Autodesk Inventor part; units mm, degrees
ref_plane "YZ Plane" through (0, 0, 0) normal (1, 0, 0) x (0, 1, 0)
ref_plane "XZ Plane" through (0, 0, 0) normal (0, 1, 0) x (-1, 0, 0)
ref_plane "XY Plane" through (0, 0, 0) normal (0, 0, 1) x (1, 0, 0)
sketch "Sketch1" plane through (0, 0, 0) normal (0, 0, 1) x (1, 0, 0)
  line L0 (0, 0) -> (161.925, 0)
  line L1 (161.925, 0) -> (161.925, 133.35)
  line L2 (161.925, 133.35) -> (0, 133.35)
  line L3 (0, 133.35) -> (0, 0)
  dimension "d0" = 161.925
  dimension "d1" = 133.35
extrude "Extrusion1" add sketch "Sketch1" along normal blind 3.175
sketch "Sketch6" plane through (0, 0, 0) normal (0, 0, -1) x (-1, 0, 0)
  circle A0 centre (-155.575, 122.2375) radius 1.5875
  circle A1 centre (-6.35, 122.2375) radius 1.5875
  circle A2 centre (-155.575, 25.4) radius 1.5875
  circle A3 centre (-6.35, 25.4) radius 1.5875
extrude "Extrusion6" cut sketch "Sketch6" against normal blind 3.175
sketch "Sketch7" plane through (0, 0, 3.175) normal (0, 0, 1) x (1, 0, 0)
  circle A0 centre (155.575, 122.2375) radius 1.5875
  circle A1 centre (6.35, 122.2375) radius 1.5875
  line L0 (9.5885, 120.3678) -> (6.35, 118.498)
  line L1 (6.35, 118.498) -> (3.1115, 120.3678)
  line L2 (3.1115, 120.3678) -> (3.1115, 124.1072)
  line L3 (3.1115, 124.1072) -> (6.35, 125.977)
  line L4 (6.35, 125.977) -> (9.5885, 124.1072)
  line L5 (9.5885, 124.1072) -> (9.5885, 120.3678)
  line L6 (158.8135, 120.3678) -> (155.575, 118.498)
  line L7 (155.575, 118.498) -> (152.3365, 120.3678)
  line L8 (152.3365, 120.3678) -> (152.3365, 124.1072)
  line L9 (152.3365, 124.1072) -> (155.575, 125.977)
  line L10 (155.575, 125.977) -> (158.8135, 124.1072)
  line L11 (158.8135, 124.1072) -> (158.8135, 120.3678)
  circle A2 centre (155.575, 25.4) radius 1.5875
  circle A3 centre (6.35, 25.4) radius 1.5875
  line L12 (9.5885, 23.5303) -> (6.35, 21.6605)
  line L13 (6.35, 21.6605) -> (3.1115, 23.5303)
  line L14 (3.1115, 23.5303) -> (3.1115, 27.2697)
  line L15 (3.1115, 27.2697) -> (6.35, 29.1395)
  line L16 (6.35, 29.1395) -> (9.5885, 27.2697)
  line L17 (9.5885, 27.2697) -> (9.5885, 23.5303)
  line L18 (158.8135, 23.5303) -> (155.575, 21.6605)
  line L19 (155.575, 21.6605) -> (152.3365, 23.5303)
  line L20 (152.3365, 23.5303) -> (152.3365, 27.2697)
  line L21 (152.3365, 27.2697) -> (155.575, 29.1395)
  line L22 (155.575, 29.1395) -> (158.8135, 27.2697)
  line L23 (158.8135, 27.2697) -> (158.8135, 23.5303)
  point P0 (9.5885, 122.2375)
  point P1 (158.8135, 122.2375)
extrude "Extrusion7" cut sketch "Sketch7" against normal blind 1.5875
sketch "Sketch11" plane through (0, 0, 3.175) normal (0, 0, 1) x (1, 0, 0)
  line L0 (161.925, 0) -> (161.925, 133.35)
  line L1 (0, 133.35) -> (0, 0)
  line L2 (0, 102.616) -> (161.925, 102.616)
  line L3 (0, 89.408) -> (161.925, 89.408)
  line L4 (0, 97.79) -> (161.925, 97.79)
  line L5 (0, 94.234) -> (161.925, 94.234)
  line L6 (0, 4.826) -> (161.925, 4.826)
  line L7 (0, 8.382) -> (161.925, 8.382)
  line L8 (0, 0) -> (161.925, 0)
  line L9 (0, 13.208) -> (161.925, 13.208)
  line L10 (0, 47.625) -> (161.925, 47.625)
  line L11 (0, 34.417) -> (161.925, 34.417)
  line L12 (0, 42.799) -> (161.925, 42.799)
  line L13 (0, 39.243) -> (161.925, 39.243)
  line L14 (161.925, 133.35) -> (0, 133.35)
  dimension "d83" = 4.826
  dimension "d84" = 3.556
  dimension "d85" = 4.826
  dimension "d86" = 4.826
  dimension "d87" = 3.556
  dimension "d88" = 4.826
  dimension "d89" = 4.826
  dimension "d90" = 3.556
  dimension "d91" = 4.826
  dimension "d96" = 30.861
  dimension "d98" = 35.56
extrude "Extrusion10" add sketch "Sketch11" along normal blind 3.302 contours L8 L1 L6 L0 | L7 L1 L9 L0 | L11 L1 L13 L0 | L12 L1 L10 L0 | L3 L1 L5 L0 | L4 L1 L2 L0
sketch "Sketch15" plane through (0, 0, 3.175) normal (0, 0, 1) x (1, 0, 0)
  line L0 (0, 102.616) -> (161.925, 102.616)
  line L1 (12.7, 120.65) -> (149.225, 120.65)
  line L2 (149.225, 120.65) -> (149.225, 102.616)
  line L3 (149.225, 102.616) -> (12.7, 102.616)
  line L4 (12.7, 102.616) -> (12.7, 120.65)
  point P0 (0, 0)
sketch "Sketch16" plane through (0, 0, 3.175) normal (0, 0, 1) x (1, 0, 0)
  line L0 (0, 47.625) -> (161.925, 47.625)
  line L1 (161.925, 89.408) -> (0, 89.408)
  line L2 (12.7, 89.408) -> (149.225, 89.408)
  line L3 (149.225, 89.408) -> (149.225, 47.625)
  line L4 (149.225, 47.625) -> (12.7, 47.625)
  line L5 (12.7, 47.625) -> (12.7, 89.408)
  point P0 (0, 0)
sketch "Sketch17" plane through (0, 0, 3.175) normal (0, 0, 1) x (1, 0, 0)
  line L0 (0, 13.208) -> (161.925, 13.208)
  line L1 (161.925, 34.417) -> (0, 34.417)
  line L2 (12.7, 34.417) -> (149.225, 34.417)
  line L3 (149.225, 34.417) -> (149.225, 13.208)
  line L4 (149.225, 13.208) -> (12.7, 13.208)
  line L5 (12.7, 13.208) -> (12.7, 34.417)
  point P0 (0, 0)
extrude "Extrusion14" cut sketch "Sketch15" against normal blind 3.175
extrude "Extrusion15" cut sketch "Sketch16" against normal blind 3.175
extrude "Extrusion16" cut sketch "Sketch17" against normal blind 3.175
fillet "Fillet5" radius 3.175 10 edges at (6.35, 102.616, 3.175) (155.575, 102.616, 3.175) (155.575, 47.625, 3.175) (6.35, 47.625, 3.175) (6.35, 13.208, 3.175) (155.575, 13.208, 3.175) (6.35, 89.408, 3.175) (155.575, 89.408, 3.175) (155.575, 34.417, 3.175) (6.35, 34.417, 3.175)
properties part number "control pod wall ROUGH"
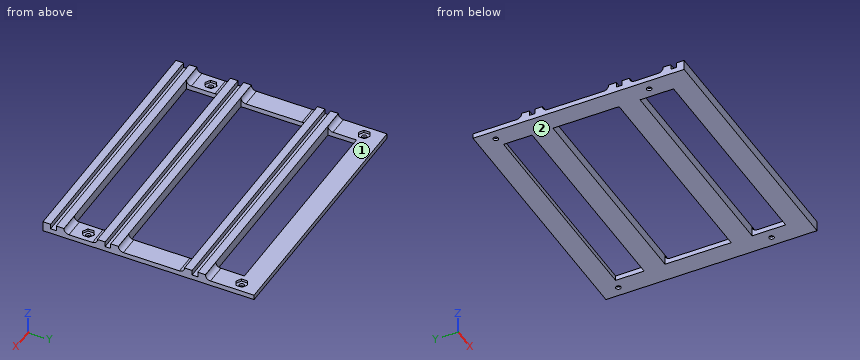
Design review of the part built by this model. Coordinates are the model's own, in mm. Face numbers are marked on the shaded views. A direction names the side the tool comes from. Round coordinates to 2 decimals unless told otherwise and drop trailing zeros. Loops run counter-clockwise (first coordinate to the right, second up) from the corner with the lowest first, then second, coordinate; pieces in that order, holes last. Notation, with made-up numbers: (17.5, 45) -> (55.5, 45) arc R23 cw to (55.5, 73) -> close; hole circle Ø5 at (70.5, -3.5). An arc over 180 degrees is marked (long way). Use one line per item in the form item = value. Start each with the question number.
Q1. We need section B-B on x = 31.5. Give the boundary of the cut face in (y, z) (3 decimals).
Q2. For pin 1 Ø3.5 at (x, y) = (155.575, 25.4) entering from +Z; pin 2 Ø1.9 at (x, z) = (55, 4) entering from +Y; pin 3 Ø2.5 at (x, y) = (155.57, 122.24) entering from -Z; pin 4 Ø1 at (x, z) = (87.5, 5.5) entering from +Y, all flat-tipped, find the tip position at first contact; note any pin that passes through.
Q3. Wall thickness on line 1 along X through (y, z) = (25.4, 1.1) (1 decimal); line 2 along Y through (x, z) = (77, 3) (3 decimals); line 3 along Y through (x, z) = (142.5, 3.5) (3 decimals): over which ranges is each line inside the solid? List them lowest first. Write a range as [from, to].
Q4. Machinability: for the marked faces 1 and 2, which of the approach directions +Z, -Z, +X, -X, +Y, -Y give a long, thin tool a straight path to every point of the face, cutting with its end or side? Answer none if there is none.
Q5. We need section A-A on y = 80. Give the boundary of the cut face in (x, z) (3 decimals), then the cut area to 3 significant figures.
Calculated:
q1.outline = (0, 0) -> (13.208, 0) -> (13.208, 6.477) -> (8.382, 6.477) -> (8.382, 3.175) -> (4.826, 3.175) -> (4.826, 6.477) -> (0, 6.477) -> close; (34.417, 0) -> (47.625, 0) -> (47.625, 6.477) -> (42.799, 6.477) -> (42.799, 3.175) -> (39.243, 3.175) -> (39.243, 6.477) -> (34.417, 6.477) -> close; (89.408, 0) -> (102.616, 0) -> (102.616, 6.477) -> (97.79, 6.477) -> (97.79, 3.175) -> (94.234, 3.175) -> (94.234, 6.477) -> (89.408, 6.477) -> close; (120.65, 0) -> (133.35, 0) -> (133.35, 3.175) -> (120.65, 3.175) -> close
q2.pin_1 = 1.59
q2.pin_2 = 133.35
q2.pin_3 = through
q2.pin_4 = 102.62
q3.line_1 = [0, 4.8], [7.9, 12.7], [149.2, 154], [157.2, 161.9]
q3.line_2 = [0, 13.208], [34.417, 47.625], [89.408, 102.616], [120.65, 133.35]
q3.line_3 = [0, 4.826], [8.382, 13.208], [34.417, 39.243], [42.799, 47.625], [89.408, 94.234], [97.79, 102.616]
q4.face_1 = +Z, +X, -X, +Y
q4.face_2 = -Z, +X, -X, +Y, -Y
q5.outline = (0, 0) -> (12.7, 0) -> (12.7, 3.175) -> (0, 3.175) -> close; (149.225, 0) -> (161.925, 0) -> (161.925, 3.175) -> (149.225, 3.175) -> close
q5.area = 80.6 mm²
